from build123d import *

# Parameters (mm, degrees)
SKETCH_1_W          = 288
SKETCH_1_H          = 101
SKETCH_1_R          = 34.5
SKETCH_1_R_2        = 1.55
EXTRUDE_1_DEPTH     = 2.5
SKETCH_2_R          = 1.5
CUT_EXTRUDE_1_DEPTH = 5
EXTRUDE_2_DEPTH     = 5
CUT_EXTRUDE_2_DEPTH = 5
CUT_EXTRUDE_3_DEPTH = 10
SKETCH_5_R          = 2
CUT_EXTRUDE_4_DEPTH = 10
SKETCH_6_R          = 1.25
CUT_EXTRUDE_5_DEPTH = 10
SKETCH_7_R          = 2
CUT_EXTRUDE_6_DEPTH = 5.5
CUT_EXTRUDE_7_DEPTH = 10
SKETCH_9_R          = 2
CUT_EXTRUDE_8_DEPTH = 10
SKETCH_10_R         = 2
CUT_EXTRUDE_9_DEPTH = 10


with BuildPart() as part:
    # Sketch 1 → Extrude 1 (new, symmetric)
    with BuildSketch(Plane.XY):
        Rectangle(SKETCH_1_W, SKETCH_1_H)
        with Locations((-54, 0)):
            Circle(SKETCH_1_R, mode=Mode.SUBTRACT)
        with Locations((-54, 37)):
            Circle(SKETCH_1_R_2, mode=Mode.SUBTRACT)
        with Locations((-35.5, 32.04293994)):
            Circle(SKETCH_1_R_2, mode=Mode.SUBTRACT)
        with Locations((-21.95706006, 18.5)):
            Circle(SKETCH_1_R_2, mode=Mode.SUBTRACT)
        with Locations((-17, 0)):
            Circle(SKETCH_1_R_2, mode=Mode.SUBTRACT)
        with Locations((-21.95706006, -18.5)):
            Circle(SKETCH_1_R_2, mode=Mode.SUBTRACT)
        with Locations((-35.5, -32.04293994)):
            Circle(SKETCH_1_R_2, mode=Mode.SUBTRACT)
        with Locations((-54, -37)):
            Circle(SKETCH_1_R_2, mode=Mode.SUBTRACT)
        with Locations((-72.5, -32.04293994)):
            Circle(SKETCH_1_R_2, mode=Mode.SUBTRACT)
        with Locations((-86.04293994, -18.5)):
            Circle(SKETCH_1_R_2, mode=Mode.SUBTRACT)
        with Locations((-91, 0)):
            Circle(SKETCH_1_R_2, mode=Mode.SUBTRACT)
        with Locations((-86.04293994, 18.5)):
            Circle(SKETCH_1_R_2, mode=Mode.SUBTRACT)
        with Locations((-72.5, 32.04293994)):
            Circle(SKETCH_1_R_2, mode=Mode.SUBTRACT)
        with Locations(Location((72.5, 32.04293994, 0), (0, 0, 180))):
            Circle(SKETCH_1_R_2, mode=Mode.SUBTRACT)
        with Locations(Location((86.04293994, 18.5, 0), (0, 0, 180))):
            Circle(SKETCH_1_R_2, mode=Mode.SUBTRACT)
        with Locations(Location((91, 0, 0), (0, 0, 180))):
            Circle(SKETCH_1_R_2, mode=Mode.SUBTRACT)
        with Locations(Location((86.04293994, -18.5, 0), (0, 0, 180))):
            Circle(SKETCH_1_R_2, mode=Mode.SUBTRACT)
        with Locations(Location((72.5, -32.04293994, 0), (0, 0, 180))):
            Circle(SKETCH_1_R_2, mode=Mode.SUBTRACT)
        with Locations(Location((54, -37, 0), (0, 0, 180))):
            Circle(SKETCH_1_R_2, mode=Mode.SUBTRACT)
        with Locations(Location((35.5, -32.04293994, 0), (0, 0, 180))):
            Circle(SKETCH_1_R_2, mode=Mode.SUBTRACT)
        with Locations(Location((21.95706006, -18.5, 0), (0, 0, 180))):
            Circle(SKETCH_1_R_2, mode=Mode.SUBTRACT)
        with Locations(Location((17, 0, 0), (0, 0, 180))):
            Circle(SKETCH_1_R_2, mode=Mode.SUBTRACT)
        with Locations(Location((21.95706006, 18.5, 0), (0, 0, 180))):
            Circle(SKETCH_1_R_2, mode=Mode.SUBTRACT)
        with Locations(Location((35.5, 32.04293994, 0), (0, 0, 180))):
            Circle(SKETCH_1_R_2, mode=Mode.SUBTRACT)
        with Locations(Location((54, 37, 0), (0, 0, 180))):
            Circle(SKETCH_1_R_2, mode=Mode.SUBTRACT)
        with Locations(Location((54, 0, 0), (0, 0, 180))):
            Circle(SKETCH_1_R, mode=Mode.SUBTRACT)
    extrude(amount=EXTRUDE_1_DEPTH, both=True)

    # Sketch 2 → Cut-Extrude 1 (cut)
    with BuildSketch(Plane.XY.offset(2.5)):
        with Locations((135, -45.5)):
            Circle(SKETCH_2_R)
        with Locations((105, -45.5)):
            Circle(SKETCH_2_R)
        with Locations((135, 24.5)):
            Circle(SKETCH_2_R)
        with Locations((105, 24.5)):
            Circle(SKETCH_2_R)
        with Locations((-105, -45.5)):
            Circle(SKETCH_2_R)
        with Locations((-135, -45.5)):
            Circle(SKETCH_2_R)
        with Locations((-105, 24.5)):
            Circle(SKETCH_2_R)
        with Locations((-135, 24.5)):
            Circle(SKETCH_2_R)
    extrude(amount=-CUT_EXTRUDE_1_DEPTH, mode=Mode.SUBTRACT)

    # Sketch 3 → Extrude 2 (add)
    with BuildSketch(Plane.XY.offset(2.5)):
        with BuildLine():
            Line((144, -50.5), (20, -50.5))
            Line((20, -50.5), (20, -55.5))
            ThreePointArc((20, -55.5), (18.5, -57), (17, -55.5))
            Line((17, -55.5), (-17, -55.5))
            ThreePointArc((-17, -55.5), (-18.5, -57), (-20, -55.5))
            Line((-20, -55.5), (-20, -50.5))
            Line((-20, -50.5), (-144, -50.5))
            Line((-144, -50.5), (-144, -56.593800871))
            ThreePointArc((-144, -56.593800871), (-142.857209562, -59.775299636), (-139.951226243, -61.502483855))
            Line((-139.951226243, -61.502483855), (-20.471229939, -84.655844628))
            ThreePointArc((-20.471229939, -84.655844628), (-19.997803382, -84.724280033), (-19.520003695, -84.747161644))
            Line((-19.520003695, -84.747161644), (19.521113953, -84.747161644))
            ThreePointArc((19.521113953, -84.747161644), (19.997818521, -84.724385042), (20.470180004, -84.656262746))
            Line((20.470180004, -84.656262746), (139.949066052, -61.557664392))
            ThreePointArc((139.949066052, -61.557664392), (142.856509449, -59.830910673), (144, -56.64856329))
            Line((144, -56.64856329), (144, -50.5))
        make_face()
    extrude(amount=-EXTRUDE_2_DEPTH)

    # Sketch 3_3 → Cut-Extrude 2 (cut)
    with BuildSketch(Plane.XY.offset(2.5)):
        Polygon((0, -50.5), (0, -45.5), (-17, -45.5), (-20, -45.5), (-20, -50.5), align=None)
        with BuildLine():
            Line((-20, -45.5), (-17, -45.5))
            ThreePointArc((-17, -45.5), (-18.5, -44), (-20, -45.5))
        make_face()
        Polygon((17, -45.5), (0, -45.5), (0, -50.5), (20, -50.5), (20, -45.5), align=None)
        with BuildLine():
            ThreePointArc((20, -45.5), (18.5, -44), (17, -45.5))
            Line((17, -45.5), (20, -45.5))
        make_face()
    extrude(amount=-CUT_EXTRUDE_2_DEPTH, mode=Mode.SUBTRACT)

    # Sketch 4 → Cut-Extrude 3 (cut)
    with BuildSketch(Plane.XY.offset(2.5)):
        Polygon((-139.951226243, -61.502483855), (139.949066052, -61.557664392), (30.752560592, -109.96050726), align=None)
    extrude(amount=-CUT_EXTRUDE_3_DEPTH, mode=Mode.SUBTRACT)

    # Sketch 5 → Cut-Extrude 4 (cut)
    with BuildSketch(Plane.XY.offset(2.5)):
        with Locations((28.453320593, -38.713035771)):
            Circle(SKETCH_5_R)
        with Locations((-28.453320593, -38.713035771)):
            Circle(SKETCH_5_R)
    extrude(amount=-CUT_EXTRUDE_4_DEPTH, mode=Mode.SUBTRACT)

    # Sketch 6 → Cut-Extrude 5 (cut)
    with BuildSketch(Plane.XY.offset(2.5)):
        with Locations((0, -40.5)):
            Circle(SKETCH_6_R)
    extrude(amount=-CUT_EXTRUDE_5_DEPTH, mode=Mode.SUBTRACT)

    # Sketch 7 → Cut-Extrude 6 (cut)
    with BuildSketch(Plane.XY.offset(2.5)):
        with Locations((90, 44)):
            Circle(SKETCH_7_R)
        with Locations((70, 44)):
            Circle(SKETCH_7_R)
    extrude(amount=-CUT_EXTRUDE_6_DEPTH, mode=Mode.SUBTRACT)

    # Sketch 8 → Cut-Extrude 7 (cut)
    with BuildSketch(Plane.XY.offset(2.5)):
        with BuildLine():
            Line((-122.656750226, 29.453887705), (-110.683185201, 38.691899695))
            ThreePointArc((-110.683185201, 38.691899695), (-109.908245536, 44.700809841), (-115.917155682, 45.475749506))
            Line((-115.917155682, 45.475749506), (-127.890720707, 36.237737517))
            ThreePointArc((-127.890720707, 36.237737517), (-128.665660372, 30.228827371), (-122.656750226, 29.453887705))
        make_face()
        with BuildLine():
            Line((-121.493437815, 21.239022322), (-132.000534722, 13.132440281))
            ThreePointArc((-132.000534722, 13.132440281), (-132.88473211, 6.276341806), (-126.028633635, 5.392144418))
            Line((-126.028633635, 5.392144418), (-115.521536728, 13.498726459))
            ThreePointArc((-115.521536728, 13.498726459), (-114.63733934, 20.354824934), (-121.493437815, 21.239022322))
        make_face()
        with BuildLine():
            Line((-114.082173129, 5.208674285), (-132.592610027, -9.072756319))
            ThreePointArc((-132.592610027, -9.072756319), (-133.583185604, -16.753715115), (-125.902226808, -17.744290693))
            Line((-125.902226808, -17.744290693), (-107.39178991, -3.462860089))
            ThreePointArc((-107.39178991, -3.462860089), (-106.401214333, 4.218098708), (-114.082173129, 5.208674285))
        make_face()
        with BuildLine():
            Line((-108.58874386, -19.943759617), (-126.661359573, -33.88739631))
            ThreePointArc((-126.661359573, -33.88739631), (-127.710476842, -42.022289495), (-119.575583656, -43.071406764))
            Line((-119.575583656, -43.071406764), (-101.502967944, -29.127770071))
            ThreePointArc((-101.502967944, -29.127770071), (-100.453850675, -20.992876886), (-108.58874386, -19.943759617))
        make_face()
        with BuildLine():
            ThreePointArc((110.683185201, 38.691899695), (109.908245536, 44.700809841), (115.917155682, 45.475749506))
            Line((115.917155682, 45.475749506), (127.890720707, 36.237737517))
            ThreePointArc((127.890720707, 36.237737517), (128.665660372, 30.228827371), (122.656750226, 29.453887705))
            Line((122.656750226, 29.453887705), (110.683185201, 38.691899695))
        make_face()
        with BuildLine():
            ThreePointArc((132.000534722, 13.132440281), (132.88473211, 6.276341806), (126.028633635, 5.392144418))
            Line((126.028633635, 5.392144418), (115.521536728, 13.498726459))
            ThreePointArc((115.521536728, 13.498726459), (114.63733934, 20.354824934), (121.493437815, 21.239022322))
            Line((121.493437815, 21.239022322), (132.000534722, 13.132440281))
        make_face()
        with BuildLine():
            ThreePointArc((132.592610027, -9.072756319), (133.583185604, -16.753715115), (125.902226808, -17.744290693))
            Line((125.902226808, -17.744290693), (107.39178991, -3.462860089))
            ThreePointArc((107.39178991, -3.462860089), (106.401214333, 4.218098708), (114.082173129, 5.208674285))
            Line((114.082173129, 5.208674285), (132.592610027, -9.072756319))
        make_face()
        with BuildLine():
            ThreePointArc((126.661359573, -33.88739631), (127.710476842, -42.022289495), (119.575583656, -43.071406764))
            Line((119.575583656, -43.071406764), (101.502967944, -29.127770071))
            ThreePointArc((101.502967944, -29.127770071), (100.453850675, -20.992876886), (108.58874386, -19.943759617))
            Line((108.58874386, -19.943759617), (126.661359573, -33.88739631))
        make_face()
    extrude(amount=-CUT_EXTRUDE_7_DEPTH, mode=Mode.SUBTRACT)

    # Sketch 9 → Cut-Extrude 8 (cut)
    with BuildSketch(Plane.XY.offset(2.5)):
        with Locations((15.453320593, -38.713035771)):
            Circle(SKETCH_9_R)
        with Locations((-15.453320593, -38.713035771)):
            Circle(SKETCH_9_R)
    extrude(amount=-CUT_EXTRUDE_8_DEPTH, mode=Mode.SUBTRACT)

    # Sketch 10 → Cut-Extrude 9 (cut)
    with BuildSketch(Plane.XY.offset(2.5)):
        with Locations((-70, 44)):
            Circle(SKETCH_10_R)
        with Locations((-90, 44)):
            Circle(SKETCH_10_R)
    extrude(amount=-CUT_EXTRUDE_9_DEPTH, mode=Mode.SUBTRACT)


solid = part.part
Source: CAD feature listing. Evaluate the final solid. Frame: model axes, mm. A direction names the side the tool comes from. Give positions to 0.01 mm unless a question says otherwise; leave off trailing zeros. Write each loop counter-clockwise with the first axis right and the second up, starting at its lowest first coordinate (ties: lowest second). Pieces come first, ordered by that corner, then holes. Notation, with made-up numbers: M 64.5,39.5 L 114.5,39.5 A29 ccw 114.5,65.5 Z; hole C 51.25,60.5 d9. An arc over 180 degrees is marked long. Return JSON: item names as keys, results as strings. Group by question number.
1) Cut plane B-B, the plane x = 79. Output: boundary loops of the cut face in (y, z).
2) Cut plane C-C, the plane z = 0.75. Give the number of separate pieces and of enclosed holes in the cut face, plus the area to 3 significant figures.
3) Cut plane D-D, the plane x = -62.5. Output: boundary loops of the cut face in (y, z).
4) Set-up query: faces 1 (the face through (0, -45.5, 0)), 2 (the face through (-2, 50.5, 0)). Return all of +Z, -Z, +X, -X, +Y, -Y with unobstructed straight access to the full face (end or side cutting, diameter ignored); none if empty.
5) Material intervals for line 1 along Y through (x, z) = (54, 0); line 2 along Y through (x, z) = (105, -1.5); line 3 along X through (y, z) = (-46.5, -1.5), sorted ascending. Write a range as [from, to].
6) Pull-direction query (Y, two-part tool) for faces 3 (the face through (-2, -5, 2.5)), 4 (the face through (-142.888, -59.738, 0.035)), 5 (the face through (110.67, -36.2, 0.04)); classes: pulls with the +Y half, pulls with the -Y half, needs draft (parallel to the pull), parting line crosses it, or undercut.
7) Cut plane A-A, the plane y = 10.5. Output: boundary loops of the cut face in (x, z), plus the area to 3 significant figures.
8) Pin query (flat end, axial travel): P1, Ø1.5, axis at x = 32, z = -2, coming from the -Y side; P2, Ø3, axis at x = 21.96, y = 18.5, coming from the +Z side. Return the tip coordinate at first contact, or that it passes through.
Recorded:
{
 "1": {"outline": "M -61.55,-2.5 L -23.77,-2.5 L -23.77,2.5 L -61.55,2.5 Z; M 23.77,-2.5 L 50.5,-2.5 L 50.5,2.5 L 23.77,2.5 Z"},
 "2": {"separate pieces": "1", "enclosed holes": "52", "area": "21,800 mm²"},
 "3": {"outline": "M -61.52,-2.5 L -33.44,-2.5 L -33.44,2.5 L -61.52,2.5 Z; M 33.44,-2.5 L 50.5,-2.5 L 50.5,2.5 L 33.44,2.5 Z"},
 "4": {"face 1": "+Z, -Z", "face 2": "+Z, -Z, +X, -X, +Y"},
 "5": {"line 1": "y = [-61.54, -38.55], [-35.45, -34.5], [34.5, 35.45], [38.55, 50.5]", "line 2": "y = [-61.55, -47], [-44, -31.83], [-18.74, 23], [26, 50.5]", "line 3": "x = [-144, -136.12], [-133.88, -106.12], [-103.88, -20], [20, 103.88], [106.12, 133.88], [136.12, 144]"},
 "6": {"face 3": "needs draft", "face 4": "pulls with the -Y half", "face 5": "undercut"},
 "7": {"outline": "M -144,-2.5 L -133.74,-2.5 L -133.74,2.5 L -144,2.5 Z; M -119.41,-2.5 L -86.86,-2.5 L -86.86,2.5 L -119.41,2.5 Z; M -21.14,-2.5 L 21.14,-2.5 L 21.14,2.5 L -21.14,2.5 Z; M 86.86,-2.5 L 119.41,-2.5 L 119.41,2.5 L 86.86,2.5 Z; M 133.74,-2.5 L 144,-2.5 L 144,2.5 L 133.74,2.5 Z", "area": "639 mm²"},
 "8": {"P1": "stops at y = -61.54", "P2": "passes through"}
}
